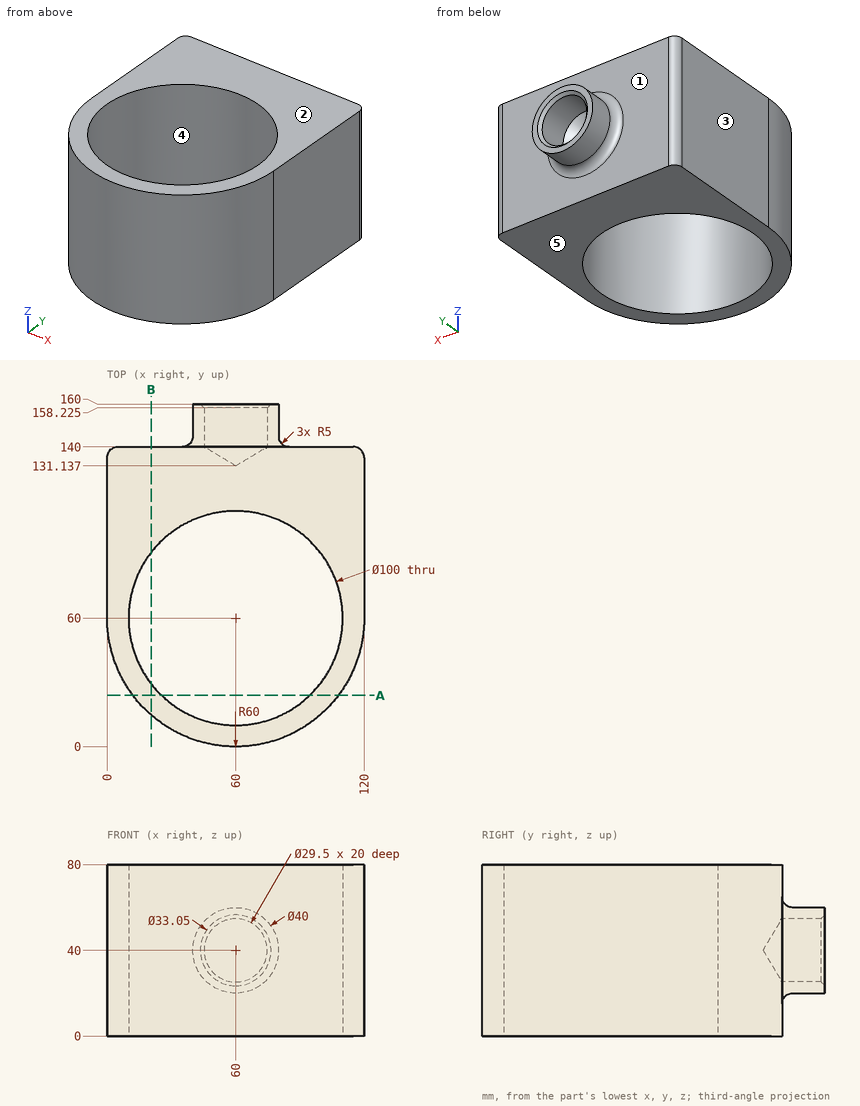
For this review, use the dimensioned drawing (mm, ordinates from the lowest corner) and the shaded views. A direction names the side the tool comes from. Give positions to 0.01 mm unless a question says otherwise; leave off trailing zeros. Order: outer loops, then holes, each group sorted by start corner. A loop starts at its lowest first (then second) coordinate and runs counter-clockwise, first axis right, second up.
1. Add section B-B, the plane x = 20.5. State the section outline as (y, z) points (1 decimal), then the cut area to 3 significant figures.
Solution:
outline: (14.8, 0) - (29.3, 0) - (29.3, 80) - (14.8, 80) - close; (90.7, 0) - (140, 0) - (140, 80) - (90.7, 80) - close
area: 5,110 mm2
2. To check wall thickness, follow L1, parallel to X at y = 145, z = 40; L2, parallel to Y at x = 60, z = 30.5 (1 decimal); L3, parallel to X at y = 39.5, z = 25 (1 decimal). State the ranges of each line that lie inside material, in increasing order.
Solution:
L1: x = 40 to 45.25, 74.75 to 80
L2: y = 0 to 10, 110 to 136.8
L3: x = 3.6 to 14.4, 105.6 to 116.4
3. Tool access review of the marked faces 1 and 2: name each direction out of +Z, -Z, +X, -X, +Y, -Y from which nothing blocks a thin tool from reaching the whole face with its end or side.
Solution:
face 1: +Y
face 2: +Z, +X, -X, +Y, -Y
4. Mouldability with a two-part tool opening along X and no side actions: class the marked faces 3, 4 and 5 as +X half, -X half, draft (parallel to the pull), parting line (faces both ways), or undercut.
Solution:
face 3: -X half
face 4: undercut
face 5: draft
5. For pin 1 Ø6 at (x, y) = (71, 107.5) entering from +Z; pin 2 Ø5 at (x, z) = (78.5, 31.5) entering from -Y; pin 3 Ø5 at (y, z) = (46, 67) entering from -X; pin 4 Ø17.5 at (x, z) = (60, 40) entering from -Y, all flat-tipped, find the tip position at first contact; note any pin that passes through.
Solution:
pin 1: stops at z = 80
pin 2: stops at y = 2.17
pin 3: stops at x = 1.11
pin 4: stops at y = 0
6. Add section A-A, the plane y = 24. State the section outline as (x, z) points.
Solution:
outline: (12, 0) - (25.3, 0) - (25.3, 80) - (12, 80) - close; (94.7, 0) - (108, 0) - (108, 80) - (94.7, 80) - close
